Work out the finished part from the listing and answer in its coordinate system (mm). A direction names the side the tool comes from. Give positions to 0.01 mm unless a question says otherwise; leave off trailing zeros. Loops run counter-clockwise (first coordinate to the right, second up) from the corner with the lowest first, then second, coordinate; pieces in that order, holes last. Notation, with made-up numbers: (-26, 84.5) -> (-4, 84.5) arc R14 cw to (-4, 95.5) -> close; hole circle Ø11 at (14, 70.5). An arc over 180 degrees is marked (long way). Answer as CSV lines item,"result". Start each with the question number.
1. Find section B-B, the plane y = 38.1. Give the vertices of the cut face in (x, z) (3 decimals).
2. Find section C-C, the plane x = 8. Give the vertices of the cut face in (y, z).
3. A tool of negligible diameter and unlimited length cuts with its end or side. For faces 1 (the face through (8, 29.6, 0.4)), 2 (the face through (30, 9.525, 0)), 3 (the face through (5, 76.2, 0)), from which of +Z, -Z, +X, -X, +Y, -Y can it reach the whole face along a straight path? Write none if from no direction.
4. Determine the mould class of faces 4 (the face through (26, 0, 0)), 5 (the face through (4.696, 55.246, -0.412)), 6 (the face through (9.525, 51, 0)) for opening direction Y: +Y half, -Y half, draft (parallel to the pull), parting line (faces both ways), or undercut.
5. Find the intervals of material crossed by line 1 along Y through (x, z) = (3.75, 0); line 2 along Z through (x, y) = (5, 38.1); line 3 along X through (y, z) = (46, -5) (3 decimals), in increasing order.
6. Find section A-A, the plane z = 0. Give the vertices of the cut face in (x, y) (3 decimals).
7. Flat-ended cylindrical pins translate along their axes: pin 1 Ø5 at (x, z) = (13.5, 17) entering from +Y (3 decimals); pin 2 Ø18.5 at (y, z) = (36, 2) entering from +X (3 decimals). Find the tip coordinate at first contact, or state that the pin passes through.
8. Find section D-D, the plane z = -18.5. Give the vertices of the cut face in (x, y) (3 decimals).
from build123d import *

# Parameters (mm, degrees)
BOSS_EXTRUDE1_DEPTH     = 25.4
SKETCH5_R               = 8.509
CUT_EXTRUDE1_DEPTH      = 3.175
CUT_EXTRUDE2_DEPTH      = 91.306287849
CUT_EXTRUDE2_DEPTH_BACK = 91.306287849
SKETCH6_R               = 6.35
F_10_24_TAPPED_HOLE1_D  = 3.7973


with BuildPart() as part:
    # Sketch2 → Boss-Extrude1 (new, symmetric)
    with BuildSketch(Plane.XY):
        Polygon((0, 0), (0, 76.2), (9.525, 76.2), (9.525, 9.525), (50.8, 9.525), (50.8, 0), align=None)
    extrude(amount=BOSS_EXTRUDE1_DEPTH, both=True)

    # Sketch5 → Cut-Extrude1 (cut)
    with BuildSketch(Plane(origin=(9.525, 0, 0), x_dir=(0, 0, -1), z_dir=(1, 0, 0))):
        with Locations(Location((0, 38.1, 0), (0, 0, 90))):
            Circle(SKETCH5_R)
    extrude(amount=-CUT_EXTRUDE1_DEPTH, mode=Mode.SUBTRACT)

    # Sketch6 → Cut-Extrude2 (cut, two sides: drawn at the far end of the back side and taken through both)
    with BuildSketch(Plane(origin=(9.525, 0, 0), x_dir=(0, 0, -1), z_dir=(1, 0, 0)).offset(-CUT_EXTRUDE2_DEPTH_BACK)):
        with Locations(Location((0, 38.1, 0), (0, 0, 90))):
            Circle(SKETCH6_R)
    extrude(amount=CUT_EXTRUDE2_DEPTH + CUT_EXTRUDE2_DEPTH_BACK, mode=Mode.SUBTRACT)

    # #10-24 Tapped Hole1 (through all)
    with Locations(Plane(origin=(9.525, 0, 0), x_dir=(0, 0, -1), z_dir=(1, 0, 0))):
        with Locations((0, 57.0992), (0, 19.1008)):
            Hole(F_10_24_TAPPED_HOLE1_D / 2)


solid = part.part
Resolved:
1,outline,"(0, -25.4) -> (9.525, -25.4) -> (9.525, -8.509) -> (6.35, -8.509) -> (6.35, -6.35) -> (0, -6.35) -> close; (0, 6.35) -> (6.35, 6.35) -> (6.35, 8.509) -> (9.525, 8.509) -> (9.525, 25.4) -> (0, 25.4) -> close"
2,outline,"(0, -25.4) -> (76.2, -25.4) -> (76.2, 25.4) -> (0, 25.4) -> close; hole circle Ø3.8 at (19.1, 0); hole circle Ø17.02 at (38.1, 0); hole circle Ø3.8 at (57.1, 0)"
3,face 1,"+X"
3,face 2,"+Z, -Z, +X, +Y"
3,face 3,"+Z, -Z, +X, -X, +Y"
4,face 4,"-Y half"
4,face 5,"undercut"
4,face 6,"draft"
5,line 1,"y = 0 to 17.2, 21 to 31.75, 44.45 to 55.2, 59 to 76.2"
5,line 2,"z = -25.4 to -6.35, 6.35 to 25.4"
5,line 3,"x = 0 to 9.525"
6,outline,"(0, 0) -> (50.8, 0) -> (50.8, 9.525) -> (9.525, 9.525) -> (9.525, 17.202) -> (0, 17.202) -> close; (0, 20.999) -> (9.525, 20.999) -> (9.525, 29.591) -> (6.35, 29.591) -> (6.35, 31.75) -> (0, 31.75) -> close; (0, 44.45) -> (6.35, 44.45) -> (6.35, 46.609) -> (9.525, 46.609) -> (9.525, 55.201) -> (0, 55.201) -> close; (0, 58.998) -> (9.525, 58.998) -> (9.525, 76.2) -> (0, 76.2) -> close"
7,pin 1,"stops at y = 9.525"
7,pin 2,"stops at x = 9.525"
8,outline,"(0, 0) -> (50.8, 0) -> (50.8, 9.525) -> (9.525, 9.525) -> (9.525, 76.2) -> (0, 76.2) -> close"
